```python
from build123d import *

# Parameters (mm, degrees)
SKETCH_1_W          = 15
SKETCH_1_H          = 10
EXTRUDE_1_DEPTH     = 10
SKETCH_1_3_W        = 15
SKETCH_1_3_H        = 10
EXTRUDE_2_DEPTH     = 20
CUT_EXTRUDE_1_DEPTH = 10


with BuildPart() as part:
    # Sketch 1 → Extrude 1 (new body)
    with BuildSketch(Plane(origin=(0, 0, 0), x_dir=(1, 0, 0), z_dir=(0, 1, 0))):
        with Locations((-7.5, 5)):
            Rectangle(SKETCH_1_W, SKETCH_1_H)
        Polygon((0, 0), (-15, 0), (-15, -10), (15, -10), (15, 0), align=None)
        with Locations((7.5, 5)):
            Rectangle(SKETCH_1_W, SKETCH_1_H)
    extrude(amount=EXTRUDE_1_DEPTH)

    # Sketch 1_3 → Extrude 2 (add)
    with BuildSketch(Plane(origin=(0, 0, 0), x_dir=(1, 0, 0), z_dir=(0, 1, 0))):
        with Locations((-7.5, 5)):
            Rectangle(SKETCH_1_3_W, SKETCH_1_3_H)
        with Locations((7.5, 5)):
            Rectangle(SKETCH_1_3_W, SKETCH_1_3_H)
    extrude(amount=EXTRUDE_2_DEPTH)

    # Sketch 2 → Cut-Extrude 1 (cut)
    with BuildSketch(Plane(origin=(0, 0, -10), x_dir=(-1, 0, 0), z_dir=(0, 0, -1))):
        Polygon((-15, 5), (0, 20), (-15, 20), align=None)
    extrude(amount=-CUT_EXTRUDE_1_DEPTH, mode=Mode.SUBTRACT)


solid = part.part
```
Input: part model. Units: mm. Frame: model coordinates. A direction names the side the tool comes from. Coordinates: 2 decimals unless noted, no trailing zeros. Write each loop counter-clockwise with the first axis right and the second up, starting at its lowest first coordinate (ties: lowest second). Pieces come first, ordered by that corner, then holes. Notation, with made-up numbers: (-0.5, 63.5) - (10.5, 63.5) arc R22 cw to (10.5, 96.5) - close; hole circle Ø10 at (1.5, 61). An arc over 180 degrees is marked (long way). Put each result on its own line as item: value. Start each with the question number.
1) Cut plane A-A (y = 8.5). Return the cut outline in (x, z), plus the area to 3 significant figures.
2) Cut plane C-C (z = -8.5). Return the cut outline in (x, y).
3) Ray query, L1, parallel to Z at x = -2.5, y = 10.25; L2, parallel to Y at x = 13.75, z = 9; L3, parallel to X at y = 18.25, z = -0.5. Return the intervals inside material, ascending.
4) Reachability of faces 1 (the face through (13, 8, 0)), 2 (the face through (-5, 15, 0)), 3 (the face through (0, 0, 0)) from +Z, -Z, +X, -X, +Y, -Y: full face, straight path, thin tool, end or side. Return the list, or none.
5) Cut plane B-B (x = 6). Return the cut outline in (y, z).
6) Contact query for flat-ended pins moving along their axis: pin 1 (8 mm diameter, centred on y = 13.5, z = -6, fed in from +X); pin 2 (1 mm diameter, centred on y = 17.5, z = -5.5, fed in from +X); pin 3 (5 mm diameter, centred on x = 1.5, y = 16.5, fed in from +Z). Output: stop coordinate, or through.
7) Cut plane D-D (y = 16.25). Return the cut outline in (x, z), plus the area to 4 significant figures.
Resolved:
1. outline: (-15, -10) - (11.5, -10) - (11.5, 0) - (15, 0) - (15, 10) - (-15, 10) - close
1. area: 565 mm2
2. outline: (-15, 0) - (15, 0) - (15, 5) - (0, 20) - (-15, 20) - close
3. L1: z = -10 to 0
3. L2: y = 0 to 10
3. L3: x = -15 to 1.75
4. face 1: -Z, +X, +Y
4. face 2: +Z, +X, -X, +Y
4. face 3: +Z, -Z, +X, -X, -Y
5. outline: (0, -10) - (14, -10) - (14, 0) - (10, 0) - (10, 10) - (0, 10) - close
6. pin 1: stops at x = 10.5
6. pin 2: stops at x = 3
6. pin 3: stops at z = 0
7. outline: (-15, -10) - (3.75, -10) - (3.75, 0) - (-15, 0) - close
7. area: 187.5 mm2
